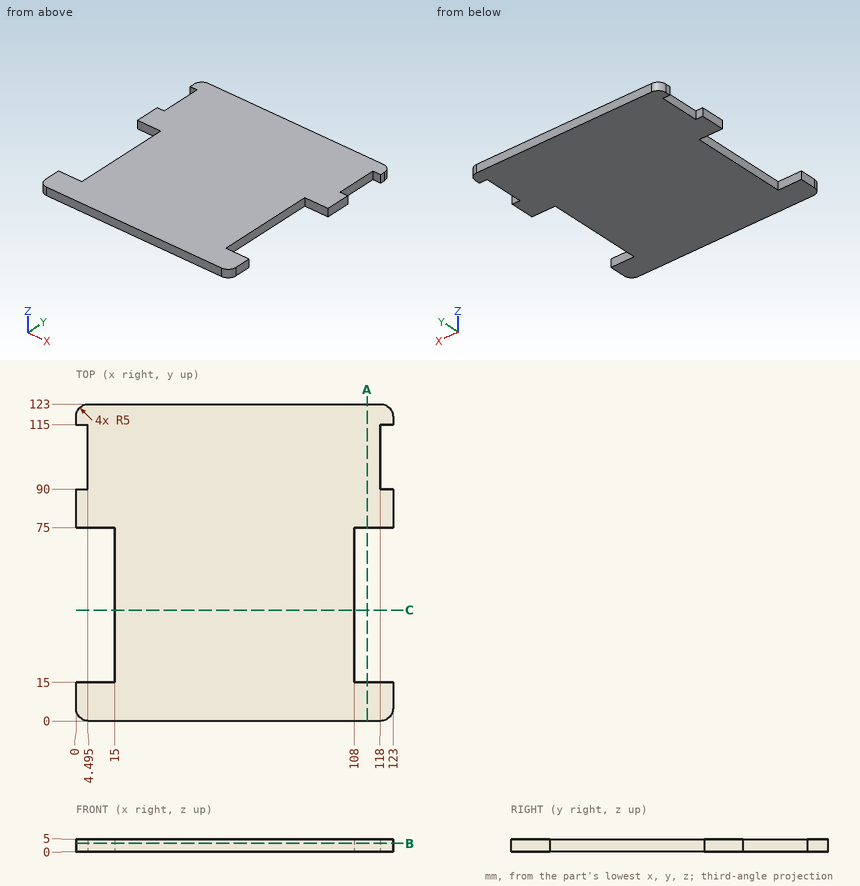
Here's the drawing with two shaded views (mm, measured from the low corner). I have some questions. Give positions to 0.01 mm unless a question says otherwise; leave off trailing zeros. Loops run counter-clockwise (first coordinate to the right, second up) from the corner with the lowest first, then second, coordinate; pieces in that order, holes last. Notation, with made-up numbers: (-19.75, 83) - (21.25, 83) arc R23 cw to (21.25, 93) - close; hole circle Ø5 at (30, 10.25). An arc over 180 degrees is marked (long way). Answer in a Markdown table with one row per item. Add a question column.
Q1. Please list where these lines run through material, in increasing order: L1, parallel to Y at x = 9.5, z = 0.4; L2, parallel to X at y = 61, z = 2.2; L3, parallel to X at y = 97, z = 3.5 (1 decimal). Write a range as from..to.
Q2. If we section it at A-A (x = 113): List the corners of the cut face in (y, z) for me.
Q3. If we section it at B-B (z = 3.3): List the corners of the cut face in (x, y) for me (1 decimal).
Q4. If we section it at C-C (y = 43): List the corners of the cut face in (x, z) for me, plus the area to 3 significant figures.
Q5. For pin 1 (1.5 mm diameter, centred on y = 55.5, z = 3.5, fed in from +X); pin 2 (2 mm diameter, centred on x = 3, z = 1.5, fed in from -Y); pin 3 (1.5 mm diameter, centred on y = 103.5, z = 2, fed in from +X), each with a flat end and sliding along its axis, tell me the tip position at first contact or that it passes through.
The answers:
| question | item | result |
|---|---|---|
| 1 | L1 | y = 0..15, 75..123 |
| 1 | L2 | x = 15..108 |
| 1 | L3 | x = 4.5..118 |
| 2 | outline | (0, 0) - (15, 0) - (15, 5) - (0, 5) - close; (75, 0) - (123, 0) - (123, 5) - (75, 5) - close |
| 3 | outline | (0, 5) arc R5 ccw to (5, 0) - (118, 0) arc R5 ccw to (123, 5) - (123, 15) - (108, 15) - (108, 75) - (123, 75) - (123, 90) - (118, 90) - (118, 115) - (123, 115) - (123, 118) arc R5 ccw to (118, 123) - (5, 123) arc R5 ccw to (0, 118) - (0, 115) - (4.5, 115) - (4.5, 90) - (0, 90) - (0, 75) - (15, 75) - (15, 15) - (0, 15) - close |
| 4 | outline | (15, 0) - (108, 0) - (108, 5) - (15, 5) - close |
| 4 | area | 465 mm^2 |
| 5 | pin 1 | stops at x = 108 |
| 5 | pin 2 | stops at y = 0.1 |
| 5 | pin 3 | stops at x = 118 |
